```python
from build123d import *

# Parameters (mm, degrees)
F1_DEPTH = 72.6
F2_R     = 7.811886
F2_R_2   = 7.792349
F3_DEPTH = 25


with BuildPart() as f1:
    # F0 (on Front) → F1 (new body)
    with BuildSketch(Plane.XZ):
        Polygon((0, 22.803508), (0, 0), (10.622752, 0), (10.622752, 10.339479), (36.400631, 10.339479), (36.400631, 0), (46.598472, 0), (46.598472, 22.803508), (36.400631, 22.803508), (36.400631, 33.001352), (10.622752, 33.001352), (10.622752, 22.803508), align=None)
    extrude(amount=F1_DEPTH)

    # F2 (on face) → F3 (cut)
    with BuildSketch(Plane.XY.offset(33.001352)):
        with Locations((23.511691, -18.15)):
            Circle(F2_R)
        with Locations((23.511691, -54.45)):
            Circle(F2_R_2)
    extrude(amount=-F3_DEPTH, mode=Mode.SUBTRACT)


solid = f1.part
```
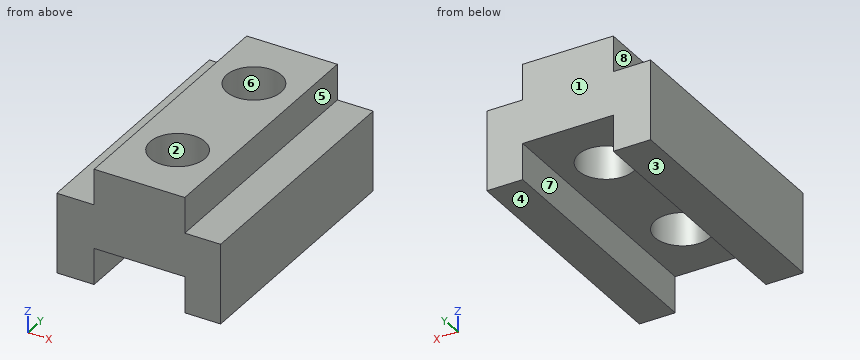
Work out the finished part from the listing and answer in its coordinate system (mm). Face numbers are marked on the shaded views. A direction names the side the tool comes from. Coordinates: 2 decimals unless noted, no trailing zeros. Order: outer loops, then holes, each group sorted by start corner. A loop starts at its lowest first (then second) coordinate and runs counter-clockwise, first axis right, second up. Notation, with made-up numbers: (70, 67) - (76, 67) arc R6 cw to (76, 77) - close; hole circle Ø3 at (10.5, 22.5). An arc over 180 degrees is marked (long way). Answer as a JSON object with one key per item and string values.
1. Each of these flat-tipped pins is pushed along its axis until it touches: P1, Ø3, axis at x = 41.5, y = -53, coming from the +Z side; P2, Ø6, axis at x = 22, y = -36, coming from the -Z side; P3, Ø12.5, axis at x = 23.51, y = -18.15, coming from the -Z side; P4, Ø5, axis at y = -29.5, z = 27.5, coming from the -X side. Where does it stop, or does it pass through?
Output values:
{"P1": "stops at z = 22.8", "P2": "stops at z = 10.34", "P3": "passes through", "P4": "stops at x = 10.62"}
2. Find section A-A on x = 23.5. Determine the outline of the cut face in (y, z).
Output values:
{"outline": "(-72.6, 10.34) - (-62.24, 10.34) - (-62.24, 33) - (-72.6, 33) - close; (-46.66, 10.34) - (-25.96, 10.34) - (-25.96, 33) - (-46.66, 33) - close; (-10.34, 10.34) - (0, 10.34) - (0, 33) - (-10.34, 33) - close"}
3. Find section D-D on y = -45.5. Determine the outline of the cut face in (x, z).
Output values:
{"outline": "(0, 0) - (10.62, 0) - (10.62, 10.34) - (36.4, 10.34) - (36.4, 0) - (46.6, 0) - (46.6, 22.8) - (36.4, 22.8) - (36.4, 33) - (10.62, 33) - (10.62, 22.8) - (0, 22.8) - close"}
4. A tool of negligible diameter and unlimited length cuts with its end or side. For the marked faces 4, 5, 6, 7 and 8, from which of +Z, -Z, +X, -X, +Y, -Y can it reach the whole face along a straight path? Write none if from no direction.
Output values:
{"face 4": "-Z, +X, -X, +Y, -Y", "face 5": "+Z, +X, +Y, -Y", "face 6": "+Z, -Z", "face 7": "-Z, +Y, -Y", "face 8": "+Z, -X, +Y, -Y"}
5. The mould has two halves that part along Y. Classify the marked faces 1, 2 and 3: +Y half, -Y half, draft (parallel to the pull), parting line (faces both ways), or undercut.
Output values:
{"face 1": "+Y half", "face 2": "undercut", "face 3": "draft"}
6. Find section B-B on y = -54.45. Determine the outline of the cut face in (x, z).
Output values:
{"outline": "(0, 0) - (10.62, 0) - (10.62, 10.34) - (15.72, 10.34) - (15.72, 33) - (10.62, 33) - (10.62, 22.8) - (0, 22.8) - close; (31.3, 10.34) - (36.4, 10.34) - (36.4, 0) - (46.6, 0) - (46.6, 22.8) - (36.4, 22.8) - (36.4, 33) - (31.3, 33) - close"}
7. Find section C-C on z = 6.5. Determine the outline of the cut face in (x, y).
Output values:
{"outline": "(0, -72.6) - (10.62, -72.6) - (10.62, 0) - (0, 0) - close; (36.4, -72.6) - (46.6, -72.6) - (46.6, 0) - (36.4, 0) - close"}
8. Consider line 1 (X direction, y = -9, z = 4.5); line 2 (Y direction, x = 30, z = 19); line 3 (Y direction, x = 26.5, z = 11.5). Determine where each line is inside the solid, lowest interval first.
Output values:
{"line 1": "x = 0 to 10.62, 36.4 to 46.6", "line 2": "y = -72.6 to -58.77, -50.13 to -22.5, -13.8 to 0", "line 3": "y = -72.6 to -61.65, -47.25 to -25.37, -10.93 to 0"}
